Model file for the job. Use its own axes, mm. Face numbers are marked on the shaded views. A direction names the side the tool comes from. Coordinates: 2 decimals unless noted, no trailing zeros. Loops run counter-clockwise (first coordinate to the right, second up) from the corner with the lowest first, then second, coordinate; pieces in that order, holes last. Notation, with made-up numbers: M 12,-9 L 64,-9 A19 ccw 64,4 Z; hole C 56,78.5 d7. An arc over 180 degrees is marked long. Write item = value, one per line. Start each with the question number.
from build123d import *

# Parameters (mm, degrees)
BOSS_EXTRUDE1_DEPTH   = 12.7
SKETCH2_R             = 8.5
CUT_EXTRUDE1_DEPTH    = 16.875
FILLET1_R             = 3.175
F_4_CLEARANCE_HOLE1_D = 2.9464
SKETCH5_W             = 24.88239846
SKETCH5_H             = 1.27
CUT_EXTRUDE2_DEPTH    = 16.875
CUT_EXTRUDE3_DEPTH    = 16.875
FILLET2_R             = 0.508


with BuildPart() as part:
    # Sketch1 → Boss-Extrude1 (new body, symmetric)
    with BuildSketch(Plane(origin=(0, 0, 0), x_dir=(0, 0, -1), z_dir=(1, 0, 0))):
        Polygon((0, 38.1), (0, 0), (15.875, 0), (15.875, 3.175), (3.175, 3.175), (3.175, 38.1), align=None)
    extrude(amount=BOSS_EXTRUDE1_DEPTH, both=True)

    # Sketch2 → Cut-Extrude1 (cut, through all)
    with BuildSketch(Plane.XY):
        with Locations((0, 25.908)):
            Circle(SKETCH2_R)
    extrude(amount=-CUT_EXTRUDE1_DEPTH, mode=Mode.SUBTRACT)

    # Fillet1
    fillet1_edges = [part.edges().sort_by_distance(p)[0] for p in [
        (12.7, 1.5875, -15.875),
        (12.7, 38.1, -1.5875),
        (-12.7, 1.5875, -15.875),
        (-12.7, 38.1, -1.5875),
    ]]
    fillet(fillet1_edges, radius=FILLET1_R)

    # #4 Clearance Hole1 (through all)
    with Locations(Plane(origin=(0, 3.175, 0), x_dir=(1, 0, 0), z_dir=(0, 1, 0))):
        with Locations((-9.525, 6.35), (0, 12.7), (9.525, 6.35)):
            Hole(F_4_CLEARANCE_HOLE1_D / 2)

    # Sketch5 → Cut-Extrude2 (cut, through all)
    with BuildSketch(Plane.XY):
        with Locations((-12.44119923, 25.908)):
            Rectangle(SKETCH5_W, SKETCH5_H)
    extrude(amount=-CUT_EXTRUDE2_DEPTH, mode=Mode.SUBTRACT)

    # Sketch6 → Cut-Extrude3 (cut, through all)
    with BuildSketch(Plane.XY):
        with BuildLine():
            Line((-9.525, 19.156703828), (-9.525, 4.7625))
            Line((-9.525, 4.7625), (9.525, 4.7625))
            Line((9.525, 4.7625), (9.525, 19.156703828))
            ThreePointArc((9.525, 19.156703828), (0, 14.233), (-9.525, 19.156703828))
        make_face()
    extrude(amount=-CUT_EXTRUDE3_DEPTH, mode=Mode.SUBTRACT)

    # Fillet2
    fillet2_edges = [part.edges().sort_by_distance(p)[0] for p in [
        (-9.525, 19.156703828, -1.5875),
        (9.525, 19.156703828, -1.5875),
        (9.525, 4.7625, -1.5875),
        (-9.525, 4.7625, -1.5875),
    ]]
    fillet(fillet2_edges, radius=FILLET2_R)


solid = part.part
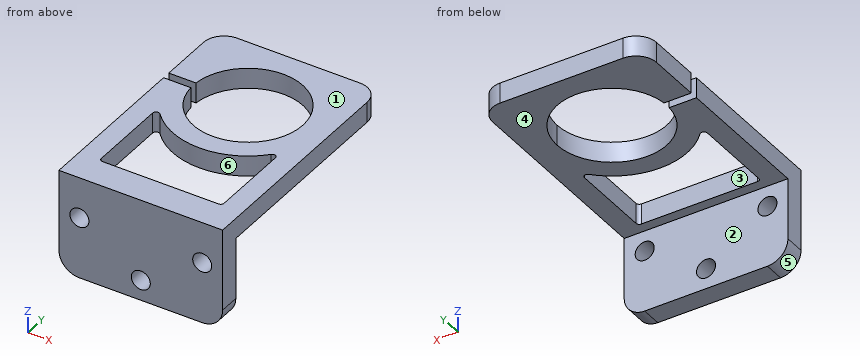
Item 1: Cut at A-A (x = 0). Give the cut face in (y, z) (1 decimal), plus the area to 3 significant figures.
Item 2: 3-axis set-ups, long thin cutter, end or side, ignore diameter. For the marked faces 1, 2 and 3: which of +Z, -Z, +X, -X, +Y, -Y reach the whole face in a straight line?
Item 3: Cut at D-D (y = 31.5). Give the cut face in (x, z) (3 decimals), plus the area to 3 significant figures.
Item 4: Pull direction X, two halves, no side cores. Call the marked faces 4, 5 and 6: +X half, -X half, draft (parallel to the pull), parting line (faces both ways), or undercut.
Item 5: Pin check, flat tips, straight feed: pin 1 Ø6 at (x, y) = (-4.5, 6.5) entering from +Z; pin 2 Ø4 at (x, z) = (-9.525, -6.35) entering from +Y (3 decimals); pin 3 Ø8 at (x, y) = (-5, 12.5) entering from -Z (3 decimals); pin 4 Ø2.5 at (x, z) = (0, -12.7) entering from +Y. Stop position of each tip, or through.
Item 6: Cut at B-B (z = -6.35). Give the cut face in (x, y) (3 decimals).
Item 7: Probe L1, parallel to X at y = 2.55, z = -6.35; L2, parallel to Z at x = 0, y = 2.55 (3 decimals); L3, parallel to X at y = 2.15, z = -12.7. List the from-to ranges inside material, lowest first.
Reported:
q1.outline = M 0,-15.9 L 3.2,-15.9 L 3.2,-14.2 L 0,-14.2 Z; M 0,-11.2 L 3.2,-11.2 L 3.2,-3.2 L 4.8,-3.2 L 4.8,0 L 0,0 Z; M 14.2,-3.2 L 17.4,-3.2 L 17.4,0 L 14.2,0 Z; M 34.4,-3.2 L 38.1,-3.2 L 38.1,0 L 34.4,0 Z
q1.area = 67.9 mm^2
q2.face_1 = +Z, +X, -X, +Y, -Y
q2.face_2 = -Z, +X, -X, +Y
q2.face_3 = +Z, -Z
q3.outline = M -12.7,-3.175 L -6.402,-3.175 L -6.402,0 L -12.7,0 Z; M 6.402,-3.175 L 12.7,-3.175 L 12.7,0 L 6.402,0 Z
q3.area = 40.0 mm^2
q4.face_4 = draft
q4.face_5 = -X half
q4.face_6 = undercut
q5.pin_1 = 0
q5.pin_2 = 3.175
q5.pin_3 = -3.175
q5.pin_4 = through
q6.outline = M -12.7,0 L -10.998,0 L -10.998,3.175 L -12.7,3.175 Z; M -8.052,0 L 8.052,0 L 8.052,3.175 L -8.052,3.175 Z; M 10.998,0 L 12.7,0 L 12.7,3.175 L 10.998,3.175 Z
q7.L1 = -12.7 to -11, -8.05 to 8.05, 11 to 12.7
q7.L2 = -15.875 to -14.173, -11.227 to 0
q7.L3 = -12.7 to -1.47, 1.47 to 12.7
